from build123d import *

# Parameters (mm, degrees)
F1_DEPTH = 63.5
F0_W     = 25.4
F0_H     = 19.05
F2_DEPTH = 25.4
F3_DEPTH = 7.9375


with BuildPart() as f1:
    # F0 (on Front) → F1 (new body, symmetric)
    with BuildSketch(Plane.XZ):
        Polygon((-38.1, -9.525), (38.1, -9.525), (38.1, 9.525), (19.05, 9.525), (-38.1, 9.525), align=None)
    extrude(amount=F1_DEPTH, both=True)

    # F0 (on Front) → F2 (join, symmetric)
    with BuildSketch(Plane.XZ):
        with BuildLine():
            Line((19.05, 9.525), (38.1, 9.525))
            Line((38.1, 9.525), (38.1, 27.0002))
            ThreePointArc((38.1, 27.0002), (42.7496798487, 38.2255201513), (53.975, 42.8752))
            Line((53.975, 42.8752), (57.15, 42.8752))
            Line((57.15, 42.8752), (57.15, 61.9252))
            Line((57.15, 61.9252), (53.975, 61.9252))
            ThreePointArc((53.975, 61.9252), (29.2792956671, 51.6959043329), (19.05, 27.0002))
            Line((19.05, 27.0002), (19.05, 9.525))
        make_face()
        with Locations((69.85, 52.4002)):
            Rectangle(F0_W, F0_H)
    extrude(amount=F2_DEPTH, both=True)

    # F0 (on Front) → F3 (join, symmetric)
    with BuildSketch(Plane.XZ):
        with BuildLine():
            add(Edge.make_bspline(
                [(-38.1, 9.525), (-38.1, 30.1610566676), (0, 61.9252), (53.975, 61.9252)],
                knots=[0, 0, 0, 0, 105.9414299745, 105.9414299745, 105.9414299745, 105.9414299745], degree=3))
            Line((-38.1, 9.525), (19.05, 9.525))
            Line((19.05, 9.525), (19.05, 27.0002))
            ThreePointArc((19.05, 27.0002), (29.2792956671, 51.6959043329), (53.975, 61.9252))
        make_face()
    extrude(amount=F3_DEPTH, both=True)

    # F0 (on Front) → F4 (revolve)
    with BuildSketch(Plane.XZ):
        Polygon((82.55, 66.675), (82.55, 61.9252), (82.55, 42.8752), (82.55, 38.1), (107.95, 38.1), (107.95, 66.675), align=None)
    revolve(axis=Axis((82.55, 0, 52.3875), (0, 0, 1)))


solid = f1.part
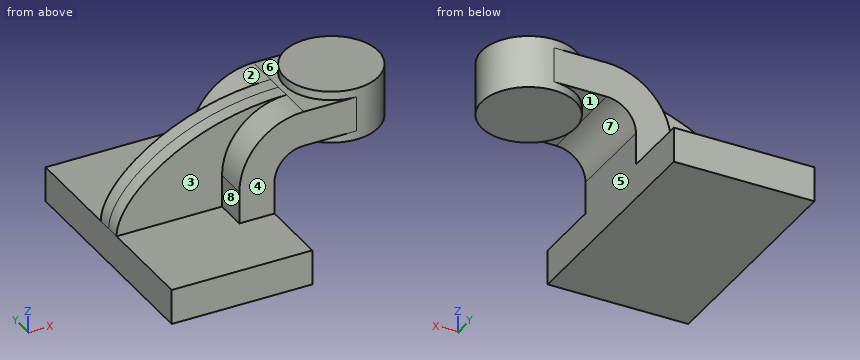
Input: part model. Units: mm. Frame: model coordinates. Face numbers are marked on the shaded views. A direction names the side the tool comes from. Coordinates: 2 decimals unless noted, no trailing zeros. Loops run counter-clockwise (first coordinate to the right, second up) from the corner with the lowest first, then second, coordinate; pieces in that order, holes last. Notation, with made-up numbers: (-39.5, -38) - (4.5, -38) arc R20 cw to (4.5, -22) - close; hole circle Ø11 at (22, 69.25). An arc over 180 degrees is marked (long way). Answer in a Markdown table with one row per item. Add a question column.
Item 1: Access query for the marked faces 1, 2, 3 and 4. Directions: +Z, -Z, +X, -X, +Y, -Y. A direction counts if a zero-diameter tool reaches every point of the face in a straight line with its end or side. Return the directions, or none.
Item 2: Section query C-C on z = -0.5. Return the cut outline in (x, y).
Item 3: Line query: line 1 along Y through (x, z) = (3, 26.5); line 2 along Z through (x, y) = (14.5, 14) (3 decimals); line 3 along Y through (x, z) = (35, 47). Output: solid intervals per line, ascending. Write a range as [from, to].
Item 4: Mould query, pull axis X, two halves, no side actions, for the marked faces 5, 6, 7 and 8. Classes: released by +X, released by -X, zero draft, split by the parting line, or undercut.
Item 5: Section query D-D on y = 17. Return the cut outline in (x, z) (3 decimals), then the cut area to 3 significant figures.
Item 6: Section query B-B on x = 59. Return the cut outline in (y, z) (3 decimals), then the cut area to 3 significant figures.
Item 7: Contact query for flat-ended pins moving along their axis: P1, Ø3, axis at y = 5.5, z = 47.5, coming from the +X side; P2, Ø3, axis at y = -31.5, z = 6.5, coming from the +X side; P3, Ø8.5, axis at y = 16, z = 15, coming from the -X side; P4, Ø15.5, axis at x = 64, z = 25.5, coming from the +Y side. Output: stop coordinate, or through.
Item 8: Section query A-A on y = -33.5. Return the cut outline in (x, z) (3 decimals), then the cut area to 3 significant figures.
Recorded:
| question | item | result |
|---|---|---|
| 1 | face 1 | -Z |
| 1 | face 2 | +Z, -X, +Y |
| 1 | face 3 | +Z, -X, -Y |
| 1 | face 4 | +Z, +X, -X, -Y |
| 2 | outline | (-38.1, -63.5) - (38.1, -63.5) - (38.1, 63.5) - (-38.1, 63.5) - close |
| 3 | line 1 | [-7.94, 7.94] |
| 3 | line 2 | [-9.525, 9.525] |
| 3 | line 3 | [-25.4, 25.4] |
| 4 | face 5 | released by +X |
| 4 | face 6 | zero draft |
| 4 | face 7 | undercut |
| 4 | face 8 | released by -X |
| 5 | outline | (-38.1, -9.525) - (38.1, -9.525) - (38.1, 27) arc R15.875 cw to (53.975, 42.875) - (63.678, 42.875) - (63.678, 38.1) - (101.422, 38.1) - (101.422, 66.675) - (63.678, 66.675) - (63.678, 61.925) - (53.975, 61.925) arc R34.925 ccw to (19.05, 27) - (19.05, 9.525) - (-38.1, 9.525) - close |
| 5 | area | 3,810 mm^2 |
| 6 | outline | (-25.4, 42.875) - (-9.516, 42.875) - (-9.516, 38.1) - (9.516, 38.1) - (9.516, 42.875) - (25.4, 42.875) - (25.4, 61.925) - (9.516, 61.925) - (9.516, 66.675) - (-9.516, 66.675) - (-9.516, 61.925) - (-25.4, 61.925) - close |
| 6 | area | 1,150 mm^2 |
| 7 | P1 | x = 107.63 |
| 7 | P2 | x = 38.1 |
| 7 | P3 | x = 19.05 |
| 7 | P4 | through |
| 8 | outline | (-38.1, -9.525) - (38.1, -9.525) - (38.1, 9.525) - (-38.1, 9.525) - close |
| 8 | area | 1,450 mm^2 |
